The model under review builds one solid part; all positions refer to its coordinate system, in mm. Face numbers are marked on the shaded views. A direction names the side the tool comes from. Coordinates: 2 decimals unless noted, no trailing zeros. Loops run counter-clockwise (first coordinate to the right, second up) from the corner with the lowest first, then second, coordinate; pieces in that order, holes last. Notation, with made-up numbers: M -27,-10.75 L -7,-10.75 A28 cw -7,7.25 Z; hole C 33,64 d11. An arc over 180 degrees is marked long. One line per item, written item: value.
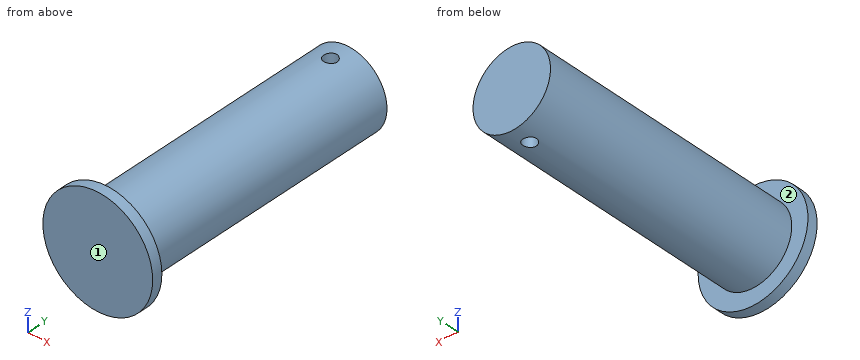
```python
from build123d import *

# Parameters (mm, degrees)
F0_R     = 19.05
F1_DEPTH = 66.675
F2_R     = 26.9875
F3_DEPTH = 5.08
F4_R     = 3.302
F5_DEPTH = 38.1


with BuildPart() as f1:
    # F0 (on Front) → F1 (new body, symmetric)
    with BuildSketch(Plane.XZ):
        Circle(F0_R)
    extrude(amount=F1_DEPTH, both=True)

    # F2 (on face) → F3 (join)
    with BuildSketch(Plane.XZ.offset(66.675)):
        Circle(F2_R)
    extrude(amount=F3_DEPTH)

    # F4 (on Top) → F5 (cut, symmetric)
    with BuildSketch(Plane.XY):
        with Locations((0, 56.769)):
            Circle(F4_R)
    extrude(amount=F5_DEPTH, both=True, mode=Mode.SUBTRACT)


solid = f1.part
```
(1) Tool access review of the marked faces 1 and 2: name each direction out of +Z, -Z, +X, -X, +Y, -Y from which nothing blocks a thin tool from reaching the whole face with its end or side.
Checks:
face 1: +Z, -Z, +X, -X, -Y
face 2: +Y
(2) Insertion check: pin 1 Ø3 at (y, z) = (-4, 10) entering from -X; pin 2 Ø2 at (x, y) = (4, -9) entering from -Z; pin 3 Ø6 at (x, y) = (-2, 14.5) entering from -Z. Each pin has a flat end and moves straight along its axis. Give the tip position at first contact, or say it passes through.
Checks:
pin 1: x = -17.05
pin 2: z = -18.81
pin 3: z = -19.05
(3) To check wall thickness, follow L1, parallel to Y at x = 0, z = -2 (3 decimals); L2, parallel to Y at x = -24, z = 7.5 (3 decimals); L3, parallel to Y at x = -0.5, z = 3.5 (3 decimals). State the ranges of each line that lie inside material, in increasing order. Write a range as [from, to].
Checks:
L1: [-71.755, 53.467], [60.071, 66.675]
L2: [-71.755, -66.675]
L3: [-71.755, 53.505], [60.033, 66.675]
(4) Add section B-B on z = 10. State the section outline as (x, y) points (3 decimals), then the cut area to 3 significant figures.
Checks:
outline: M -25.066,-71.755 L 25.066,-71.755 L 25.066,-66.675 L 16.214,-66.675 L 16.214,66.675 L -16.214,66.675 L -16.214,-66.675 L -25.066,-66.675 Z; hole C 0,56.769 d6.604
area: 4,540 mm^2
(5) Add section D-D on y = -12. State the section outline as (x, z) points, then the cut area to 3 significant figures.
Checks:
outline: C 0,0 d38.1
area: 1,140 mm^2
